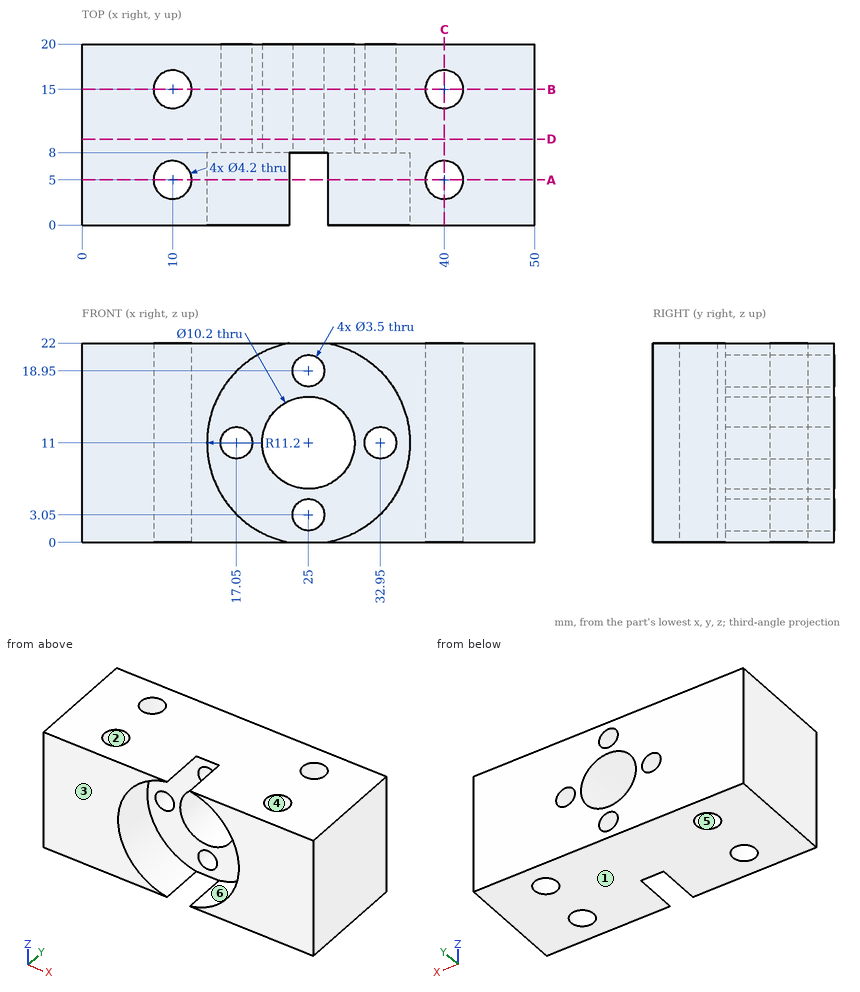
Input: dimensioned drawing with shaded views. Units: mm. Origin: part minimum x, y, z. A direction names the side the tool comes from. Coordinates: 2 decimals unless noted, no trailing zeros. Order: outer loops, then holes, each group sorted by start corner. A loop starts at its lowest first (then second) coordinate and runs counter-clockwise, first axis right, second up.
1. Access query for the marked faces 5 and 6. Directions: +Z, -Z, +X, -X, +Y, -Y. A direction counts if a zero-diameter tool reaches every point of the face in a straight line with its end or side. Return the directions, or none.
Checked values:
face 5: +Z, -Z
face 6: -Y
2. Cut plane D-D, the plane y = 9.5. Return loops of the section in (x, z).
Checked values:
outline: (0, 0) - (50, 0) - (50, 22) - (0, 22) - close; hole circle Ø3.5 at (17.05, 11); hole circle Ø10.2 at (25, 11); hole circle Ø3.5 at (25, 3.05); hole circle Ø3.5 at (25, 18.95); hole circle Ø3.5 at (32.95, 11)
3. Ray query, line 1 along Y through (x, z) = (40, 18.25); line 2 along Z through (x, y) = (25, 16.25); line 3 along X through (y, z) = (9, 12.5). Return the intervals inside material, ascending.
Checked values:
line 1: y = 0 to 2.9, 7.1 to 12.9, 17.1 to 20
line 2: z = 0 to 1.3, 4.8 to 5.9, 16.1 to 17.2, 20.7 to 22
line 3: x = 0 to 16.15, 17.95 to 20.13, 29.87 to 32.05, 33.85 to 50
4. Cut plane B-B, the plane y = 15. Return loops of the section in (x, z).
Checked values:
outline: (0, 0) - (7.9, 0) - (7.9, 22) - (0, 22) - close; (12.1, 0) - (37.9, 0) - (37.9, 22) - (12.1, 22) - close; (42.1, 0) - (50, 0) - (50, 22) - (42.1, 22) - close; hole circle Ø3.5 at (17.05, 11); hole circle Ø10.2 at (25, 11); hole circle Ø3.5 at (25, 3.05); hole circle Ø3.5 at (25, 18.95); hole circle Ø3.5 at (32.95, 11)
5. Cut plane A-A, the plane y = 5. Return loops of the section in (x, z), plus the area to 3 significant figures.
Checked values:
outline: (0, 0) - (7.9, 0) - (7.9, 22) - (0, 22) - close; (12.1, 0) - (22.89, 0) arc R11.2 cw to (22.89, 22) - (12.1, 22) - close; (27.11, 0) - (37.9, 0) - (37.9, 22) - (27.11, 22) arc R11.2 cw to start; (42.1, 0) - (50, 0) - (50, 22) - (42.1, 22) - close
area: 522 mm2
6. Contact query for flat-ended pins moving along their axis: P1, Ø1, axis at y = 2.5, z = 18, coming from the -X side; P2, Ø11.5, axis at x = 25, z = 11, coming from the -Y side. Output: stop coordinate, or through.
Checked values:
P1: stops at x = 0
P2: stops at y = 8
7. Cut plane C-C, the plane x = 40. Return loops of the section in (y, z), plus the area to 3 significant figures.
Checked values:
outline: (0, 0) - (2.9, 0) - (2.9, 22) - (0, 22) - close; (7.1, 0) - (12.9, 0) - (12.9, 22) - (7.1, 22) - close; (17.1, 0) - (20, 0) - (20, 22) - (17.1, 22) - close
area: 255 mm2
8. Draft query along Y for the marked faces 1, 2, 3 and 4. Return one class per face: +Y half, -Y half, draft (parallel to the pull), parting line (faces both ways), or undercut.
Checked values:
face 1: draft
face 2: undercut
face 3: -Y half
face 4: undercut
